```python
from build123d import *

# Parameters (mm, degrees)
F0_W      = 1618
F0_H      = 45
F1_DEPTH  = 22.5
F3_D      = 11
F3_DEPTH  = 27
F3_TIP    = 3.3047334047
F5_DEPTH  = 15
F7_DEPTH  = 15
F8_R      = 9
F9_DEPTH  = 30
F11_D     = 3.5
F11_DEPTH = 30
F11_TIP   = 1.0515060833


with BuildPart() as f1:
    # F0 (on Right) → F1 (new body, symmetric)
    with BuildSketch(Plane.YZ):
        with Locations((809, 0)):
            Rectangle(F0_W, F0_H)
    extrude(amount=F1_DEPTH, both=True)

    # F3
    with Locations(Plane.XZ):
        with Locations((0, 0)):
            Hole(F3_D / 2, depth=F3_DEPTH)
            with Locations((0, 0, -(F3_DEPTH + F3_TIP / 2))):  # 118° drill point
                Cone(0, F3_D / 2, F3_TIP, mode=Mode.SUBTRACT)

    # F4 (on face) → F5 (cut)
    with BuildSketch(Plane.YZ.offset(22.5)):
        Polygon((1618, -22.5), (1618, 22.5), (1573, -22.5), align=None)
    extrude(amount=-F5_DEPTH, mode=Mode.SUBTRACT)

    # F6 (on face) → F7 (cut)
    with BuildSketch(Plane(origin=(-22.5, 0, 0), x_dir=(0, -1, 0), z_dir=(-1, 0, 0))):
        Polygon((-1573, -22.5), (-1618, 22.5), (-1618, -22.5), align=None)
    extrude(amount=-F7_DEPTH, mode=Mode.SUBTRACT)

    # F8 (on face) → F9 (cut)
    with BuildSketch(Plane(origin=(-22.5, 0, 0), x_dir=(0, -1, 0), z_dir=(-1, 0, 0))):
        with Locations((-200, 0)):
            Circle(F8_R)
        with Locations((-500, 0)):
            Circle(F8_R)
        with Locations((-800, 0)):
            Circle(F8_R)
        with Locations((-1100, 0)):
            Circle(F8_R)
        with Locations((-1400, 0)):
            Circle(F8_R)
    extrude(amount=-F9_DEPTH, mode=Mode.SUBTRACT)

    # F11
    with Locations(Plane(origin=(0, 0, -22.5), x_dir=(1, 0, 0), z_dir=(0, 0, -1))):
        with Locations((10, -1548), (10, -1508), (10, -1468), (-10, -1468), (-10, -1508), (-10, -1548)):
            Hole(F11_D / 2, depth=F11_DEPTH)
            with Locations((0, 0, -(F11_DEPTH + F11_TIP / 2))):  # 118° drill point
                Cone(0, F11_D / 2, F11_TIP, mode=Mode.SUBTRACT)


solid = f1.part
```
CAD build for the part. Positions are in the model's coordinates, mm. A direction names the side the tool comes from. Round coordinates to 2 decimals unless told otherwise and drop trailing zeros.
Item 1: Probe line 1 along X through (y, z) = (1468, -10); line 2 along Y through (x, z) = (10, -14.5); line 3 along Y through (x, z) = (10, -1). List the from-to ranges inside material, lowest first.
Item 2: Pin check, flat tips, straight feed: pin 1 (3 mm diameter, centred on x = 10, y = 1548, fed in from -Z); pin 2 (16 mm diameter, centred on y = 200, z = 0, fed in from -X). Stop position of each tip, or through.
Item 3: Tool access for faces 1 (the face through (-22.5, 798, 10)), 2 (the face through (-15.1, 1595.2, -0.3)), 3 (the face through (7.5, 1605, -10)): list every direction of +Z, -Z, +X, -X, +Y, -Y with a clear straight run to the whole face (end or side of a thin tool).
Reported:
1. line 1: x = -22.5 to -11.75, -8.25 to 8.25, 11.75 to 22.5
1. line 2: y = 0 to 1466.25, 1469.75 to 1506.25, 1509.75 to 1546.25, 1549.75 to 1581
1. line 3: y = 0 to 1466.25, 1469.75 to 1506.25, 1509.75 to 1546.25, 1549.75 to 1594.5
2. pin 1: stops at z = 7.65
2. pin 2: stops at x = 7.5
3. face 1: +Z, -Z, -X, +Y, -Y
3. face 2: -Z, -X, +Y
3. face 3: -Z, +X, +Y
